Check sheet for the modelled part. Datum: model origin and axes. Units: mm. Face numbers are marked on the shaded views. A direction names the side the tool comes from. Coordinates: 2 decimals unless noted, no trailing zeros. Loops run counter-clockwise (first coordinate to the right, second up) from the corner with the lowest first, then second, coordinate; pieces in that order, holes last. Notation, with made-up numbers: (-9, -37.5) - (30, -37.5) arc R35 ccw to (30, -5.5) - close; hole circle Ø5 at (0, 85). An arc over 180 degrees is marked (long way). Write each question's results on one line, items separated by ' | '. Start each with the question number.
1. Cross-section at C-C (z = -25). Record the cut outline in (x, y) (3 decimals), and give its area (3 significant figures).
2. Thickness scan on line 1 (X direction, y = 6.25, z = 12.5); line 2 (X direction, y = 8, z = -4); line 3 (Z direction, x = -7, y = 1.5). Record the ranges inside material, lowest first. Write a range as [from, to].
3. Cross-section at A-A (x = 0). Give the number of separate pieces and of enclosed holes in the cut face, and give its area (3 significant figures).
4. Gauge pin test, flat ends, axial feed: P1, Ø4, axis at x = 28, y = 5.5, coming from the +Z side; P2, Ø2.5, axis at x = 33, y = 2.5, coming from the -Z side; P3, Ø2, axis at x = -21, y = 5, coming from the -Z side. Record the tip position at first contact, or that the pin passes through.
5. Tool access check on the marked faces 4 and 5. Record the directions out of +Z, -Z, +X, -X, +Y, -Y that give a thin tool (end or side, any length) a straight path to the whole face; none if there is none.
6. Draft check along Z on the marked faces 1, 2 and 3. Enter one of: released by +Z, released by -Z, zero draft, split by the parting line, or undercut.
7. Cross-section at B-B (z = 12.5). Record the cut outline in (x, y) (3 decimals).
```python
from build123d import *

# Parameters (mm, degrees)
BASEPLATE_SKETCH_R   = 2.1
BASEPLATE_SKETCH_R_2 = 6.25
BOSS_EXTRUDE1_DEPTH  = 9.525
SKETCH2_R            = 2.25
CUT_EXTRUDE1_DEPTH   = 25
CIRPATTERN1_COUNT    = 3
SKETCH3_R            = 1.25
CUT_EXTRUDE2_DEPTH   = 9.525


with BuildPart() as part:
    # Baseplate Sketch → Boss-Extrude1 (new body)
    with BuildSketch(Plane(origin=(0, 0, 0), x_dir=(1, 0, 0), z_dir=(0, 1, 0))):
        with BuildLine():
            ThreePointArc((17.5, 30.310889132), (0, 35), (-17.5, 30.310889132))
            Line((-17.5, 30.310889132), (-15, 25.980762114))
            ThreePointArc((-15, 25.980762114), (-25.980762114, 15), (-30, 0))
            Line((-30, 0), (-35, 0))
            ThreePointArc((-35, 0), (-30.310889132, -17.5), (-17.5, -30.310889132))
            Line((-17.5, -30.310889132), (-15, -25.980762114))
            ThreePointArc((-15, -25.980762114), (0, -30), (15, -25.980762114))
            Line((15, -25.980762114), (17.5, -30.310889132))
            ThreePointArc((17.5, -30.310889132), (30.310889132, -17.5), (35, 0))
            Line((35, 0), (30, 0))
            ThreePointArc((30, 0), (25.980762114, 15), (15, 25.980762114))
            Line((15, 25.980762114), (17.5, 30.310889132))
        make_face()
        with Locations(Location((0, 25, 0), (0, 0, 90))):
            Circle(BASEPLATE_SKETCH_R, mode=Mode.SUBTRACT)
        with Locations(Location((-21.650635095, -12.5, 0), (0, 0, 90))):
            Circle(BASEPLATE_SKETCH_R, mode=Mode.SUBTRACT)
        with Locations(Location((0, 0, 0), (0, 0, 90))):
            Circle(BASEPLATE_SKETCH_R_2, mode=Mode.SUBTRACT)
        with Locations(Location((21.650635095, -12.5, 0), (0, 0, 90))):
            Circle(BASEPLATE_SKETCH_R, mode=Mode.SUBTRACT)
    extrude(amount=BOSS_EXTRUDE1_DEPTH)

    # Sketch2 → Cut-Extrude1 (cut)
    with BuildSketch(Plane.XY.offset(40)):
        with Locations((0, 4.7625)):
            Circle(SKETCH2_R)
    cut_extrude1 = extrude(amount=-CUT_EXTRUDE1_DEPTH, mode=Mode.SUBTRACT)

    # CirPattern1: Cut-Extrude1 ×3 about axis
    cirpattern1_axis = Axis((0, 0, 0), (0, 1, 0))
    for i in range(1, CIRPATTERN1_COUNT):
        add(cut_extrude1.rotate(cirpattern1_axis, i * 360 / CIRPATTERN1_COUNT), mode=Mode.SUBTRACT)

    # Sketch3 → Cut-Extrude2 (cut)
    with BuildSketch(Plane(origin=(0, 9.525, 0), x_dir=(1, 0, 0), z_dir=(0, 1, 0))):
        with Locations(Location((-8.127648415, -4.6925, 0), (0, 0, 270))):
            Circle(SKETCH3_R)
        with Locations(Location((0, -9.385, 0), (0, 0, 270))):
            Circle(SKETCH3_R)
        with Locations(Location((-8.127648415, 4.6925, 0), (0, 0, 270))):
            Circle(SKETCH3_R)
        with Locations(Location((0, 9.385, 0), (0, 0, 270))):
            Circle(SKETCH3_R)
        with Locations(Location((8.127648415, 4.6925, 0), (0, 0, 270))):
            Circle(SKETCH3_R)
        with Locations(Location((8.127648415, -4.6925, 0), (0, 0, 270))):
            Circle(SKETCH3_R)
    extrude(amount=-CUT_EXTRUDE2_DEPTH, mode=Mode.SUBTRACT)


solid = part.part
```
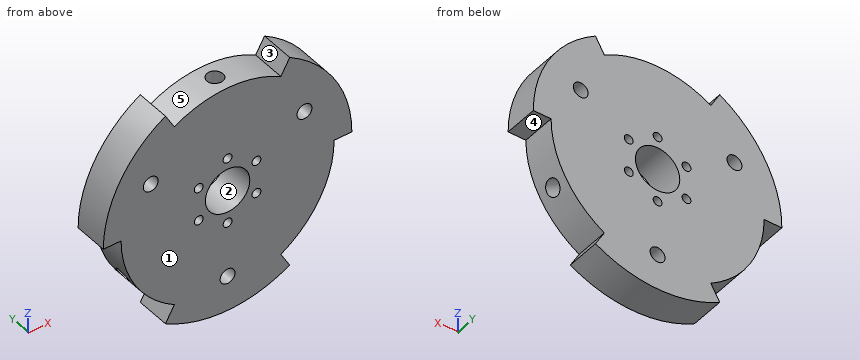
Established:
1) outline: (-16.583, 0) - (-2.1, 0) - (-2.1, 9.525) - (-16.583, 9.525) - close; (2.1, 0) - (16.583, 0) - (16.583, 9.525) - (2.1, 9.525) - close | area: 276 mm^2
2) line 1: [-32.69, -23.75], [-19.55, 19.55], [23.75, 32.69] | line 2: [-29.73, -9.17], [-7.09, -4.8], [4.8, 7.09], [9.17, 29.73] | line 3: [-34.29, -5.23], [-4.15, 4.15], [5.23, 29.17]
3) separate pieces: 5 | enclosed holes: 0 | area: 345 mm^2
4) P1: z = 23.43 | P2: z = 0 | P3: z = -22.36
5) face 4: -Z, +X, +Y, -Y | face 5: +Z, +Y, -Y
6) face 1: zero draft | face 2: undercut | face 3: released by +Z
7) outline: (-32.692, 0) - (-23.751, 0) - (-23.751, 9.525) - (-32.692, 9.525) - close; (-19.551, 0) - (19.551, 0) - (19.551, 9.525) - (-19.551, 9.525) - close; (23.751, 0) - (32.692, 0) - (32.692, 9.525) - (23.751, 9.525) - close
